Input: part model. Units: mm. Frame: model coordinates. Give positions to 0.01 mm unless a question says otherwise; leave off trailing zeros. Write each loop counter-clockwise with the first axis right and the second up, starting at its lowest first coordinate (ties: lowest second). Pieces come first, ordered by that corner, then holes. Notation, with made-up numbers: (-31.75, 75.5) - (11.25, 75.5) arc R27 ccw to (11.25, 96.5) - close; hole circle Ø11 at (69.25, 36). An arc over 180 degrees is marked (long way). Answer as CSV lines item,"result".
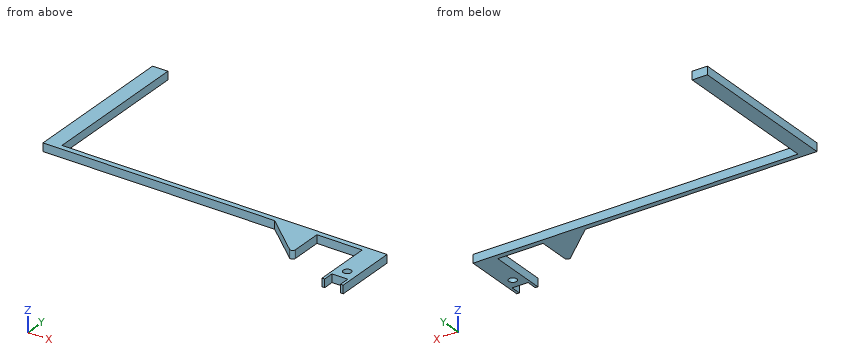
Autodesk Inventor part; units mm, degrees
ref_plane "YZ Plane" through (0, 0, 0) normal (1, 0, 0) x (0, 1, 0)
ref_plane "XZ Plane" through (0, 0, 0) normal (0, 1, 0) x (-1, 0, 0)
ref_plane "XY Plane" through (0, 0, 0) normal (0, 0, 1) x (1, 0, 0)
sketch "Sketch1" plane through (0, 0, 0) normal (0, 0, 1) x (1, 0, 0)
  line L0 (0, 0) -> (3.175, 0)
  line L1 (3.175, 0) -> (3.175, 12.7)
  line L2 (3.175, 12.7) -> (22.225, 12.7)
  line L3 (22.225, 12.7) -> (22.225, 0)
  line L4 (22.225, 0) -> (25.4, 0)
  circle A0 centre (12.7, 25.4) radius 4.7815
  line L5 (25.4, 0) -> (25.4, 76.2)
  line L6 (25.4, 76.2) -> (-384.175, 76.2)
  line L7 (0, 69.85) -> (0, 0)
  line L8 (-54.61, 69.85) -> (-54.61, 32.397)
  line L9 (-59.8758, 30.0075) -> (-105.41, 69.85)
  ellipse E0 centre (-26.9408, 50.8) end of major axis (0, 50.8) minor radius 19.05
  arc A1 (-59.8758, 30.0075) -> (-54.61, 32.397) centre (-57.785, 32.397) ccw
  line L10 (-384.175, 69.85) -> (-105.41, 69.85)
  line L11 (-54.61, 69.85) -> (0, 69.85)
  line L12 (-384.175, 69.85) -> (-384.175, 260.35)
  line L13 (-384.175, 260.35) -> (-365.76, 260.35)
  line L14 (-365.76, 260.35) -> (-365.76, 76.2)
  point P0 (-54.61, 25.4)
  dimension "d15" = 26.9408
  dimension "d16" = 19.05
  dimension "d0" = 3.175
  dimension "d1" = 12.7
  dimension "d2" = 19.05
  dimension "d3" = 3.175
  dimension "d4" = 12.7
  dimension "d6" = 9.5631
  dimension "d7" = 12.7
  dimension "d8" = 76.2
  dimension "d9" = 409.575
  dimension "d10" = 6.35
  dimension "d11" = 384.175
  dimension "d13" = 50.8
  dimension "d14" = 54.61
  dimension "d17" = 44.45
  dimension "d18" = 3.175
  dimension "d21" = 190.5
  dimension "d22" = 18.415
  dimension "d24" = 9.525
  dimension "d25" = 184.15
extrude "Extrusion1" add sketch "Sketch1" along normal blind 9.8425 contours L7 L11 L8 A1 L9 L10 L12 L6 L5 L4 L3 L2 L1 L0 | L6 L12 L13 L14
properties part number "Left Climber Hook"
Item 1: Contact query for flat-ended pins moving along their axis: pin 1 (3 mm diameter, centred on x = -138, z = 6.5, fed in from +Y); pin 2 (3 mm diameter, centred on x = 9, z = 2.5, fed in from -Y); pin 3 (5 mm diameter, centred on x = -239, z = 5, fed in from -Y). Output: stop coordinate, or through.
The answers:
pin 1,"y = 76.2"
pin 2,"y = 12.7"
pin 3,"y = 69.85"
Item 2: Cut plane D-D on x = -134.5. Return the cut outline in (y, z), plus the area to 3 significant figures.
The answers:
outline,"(69.85, 0) - (76.2, 0) - (76.2, 9.84) - (69.85, 9.84) - close"
area,"62.5 mm²"
Item 3: Cut plane C-C on y = 125. Return the cut outline in (x, z) (1 decimal).
The answers:
outline,"(-384.2, 0) - (-365.8, 0) - (-365.8, 9.8) - (-384.2, 9.8) - close"
Item 4: Cut plane B-B on x = 12.7. Return the cut outline in (y, z).
The answers:
outline,"(12.7, 0) - (20.62, 0) - (20.62, 9.84) - (12.7, 9.84) - close; (30.18, 0) - (76.2, 0) - (76.2, 9.84) - (30.18, 9.84) - close"
Item 5: Ray query, line 1 (Y direction, x = 12.7, z = 2.75); line 2 (Y direction, x = -276, z = 6.75); line 3 (X direction, y = 114.5, z = 5.5) (3 decimals). Return the intervals inside material, ascending. Write a range as from..to.
The answers:
line 1,"12.7..20.62, 30.18..76.2"
line 2,"69.85..76.2"
line 3,"-384.175..-365.76"
